Input: dimensioned drawing with shaded views. Units: mm. Origin: part minimum x, y, z. A direction names the side the tool comes from. Give positions to 0.01 mm unless a question says otherwise; leave off trailing zeros. Write each loop counter-clockwise with the first axis right and the second up, starting at its lowest first coordinate (ties: lowest second). Pieces come first, ordered by that corner, then holes.
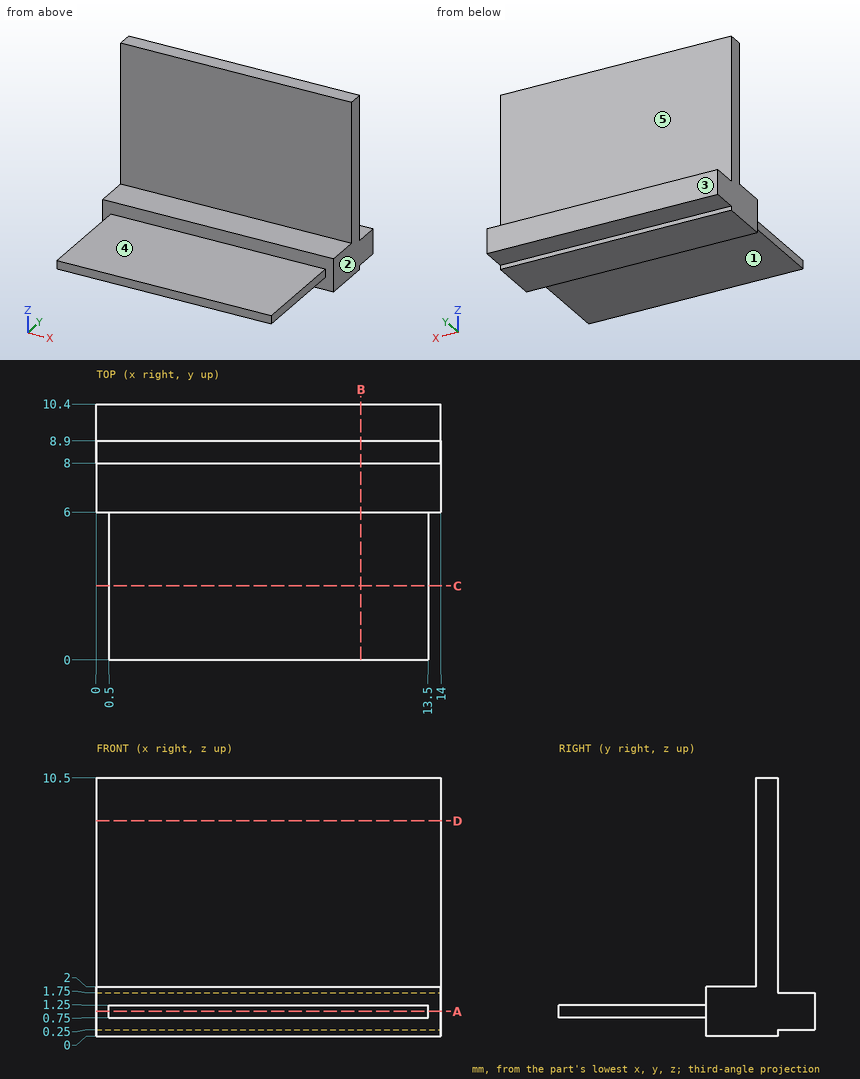
Item 1: Pin query (flat end, axial travel): pin 1 (3 mm diameter, centred on y = 1.5, z = 4, fed in from +X) (3 decimals); pin 2 (1 mm diameter, centred on x = 2.5, z = 5, fed in from +Y); pin 3 (1.5 mm diameter, centred on x = 6.5, y = 3, fed in from -Z); pin 4 (0.8 mm diameter, centred on x = 10, y = 10, fed in from +Z). Return the tip coordinate at first contact, or that it passes through.
Item 2: Ray query, line 1 (Y direction, x = 2.25, z = 7.25); line 2 (Z direction, x = 2.25, y = 7.5); line 3 (Z direction, x = 9.75, y = 4.5). Return the intervals inside material, ascending.
Item 3: Section B-B (x = 10.75). Return loops of the section in (y, z), and give its area (3 significant figures).
Item 4: Set-up query: the marked faces 1, 2, 3, 4 and 5. Return all of +Z, -Z, +X, -X, +Y, -Y with unobstructed straight access to the full face (end or side cutting, diameter ignored); none if empty.
Item 5: Section C-C (y = 3). Return loops of the section in (x, z), and give its area (3 significant figures).
Item 6: Section A-A (z = 1). Return loops of the section in (x, y), and give its area (3 significant figures).
Item 7: Section D-D (z = 8.75). Return loops of the section in (x, y).
Solved:
1. pin 1: passes through
1. pin 2: stops at y = 8.9
1. pin 3: stops at z = 0.75
1. pin 4: stops at z = 1.75
2. line 1: y = 8 to 8.9
2. line 2: z = 0 to 2
2. line 3: z = 0.75 to 1.25
3. outline: (0, 0.75) - (6, 0.75) - (6, 0) - (8.9, 0) - (8.9, 0.25) - (10.4, 0.25) - (10.4, 1.75) - (8.9, 1.75) - (8.9, 10.5) - (8, 10.5) - (8, 2) - (6, 2) - (6, 1.25) - (0, 1.25) - close
3. area: 18.7 mm2
4. face 1: -Z, +X, -X, -Y
4. face 2: +Z, -Z, +X, +Y, -Y
4. face 3: +Z, -Z, +X, -X, +Y
4. face 4: +Z, +X, -X, -Y
4. face 5: +Z, +X, -X, +Y
5. outline: (0.5, 0.75) - (13.5, 0.75) - (13.5, 1.25) - (0.5, 1.25) - close
5. area: 6.50 mm2
6. outline: (0, 6) - (0.5, 6) - (0.5, 0) - (13.5, 0) - (13.5, 6) - (14, 6) - (14, 10.4) - (0, 10.4) - close
6. area: 140 mm2
7. outline: (0, 8) - (14, 8) - (14, 8.9) - (0, 8.9) - close
